Here's how the part is built. I have some questions about the finished solid (model axes, mm). Face numbers are marked on the shaded views. Round coordinates to 2 decimals unless told otherwise and drop trailing zeros. Write each loop counter-clockwise with the first axis right and the second up, starting at its lowest first coordinate (ties: lowest second). Pieces come first, ordered by that corner, then holes. Notation, with made-up numbers: (69.5, -15.5) -> (93.5, -15.5) arc R38 cw to (93.5, 22.5) -> close; hole circle Ø2 at (-26, -6). An arc over 180 degrees is marked (long way). Answer as CSV lines item,"result".
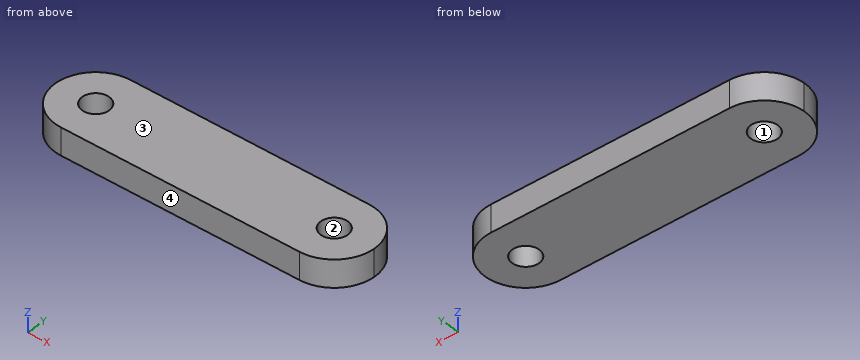
```python
from build123d import *

# Parameters (mm, degrees)
F1_DEPTH = 10
F2_R     = 5
F3_DEPTH = 25


with BuildPart() as f1:
    # F0 (on Top) → F1 (new body)
    with BuildSketch(Plane.XY):
        with BuildLine():
            ThreePointArc((60, 0), (55.606602, 10.606602), (45, 15))
            Line((45, 15), (-45, 15))
            ThreePointArc((-45, 15), (-55.606602, 10.606602), (-60, 0))
            ThreePointArc((-60, 0), (-55.606602, -10.606602), (-45, -15))
            Line((-45, -15), (45, -15))
            ThreePointArc((45, -15), (55.606602, -10.606602), (60, 0))
        make_face()
    extrude(amount=F1_DEPTH)

    # F2 (on face) → F3 (cut)
    with BuildSketch(Plane.XY.offset(10)):
        with Locations((-45, 0)):
            Circle(F2_R)
        with Locations((45, 0)):
            Circle(F2_R)
    extrude(amount=-F3_DEPTH, mode=Mode.SUBTRACT)


solid = f1.part
```
1. Suppose I cut it at A-A on z = 6.5. Please give me the cut outline in (x, y).
Numbers:
outline,"(-60, 0) arc R15 ccw to (-45, -15) -> (45, -15) arc R15 ccw to (60, 0) arc R15 ccw to (45, 15) -> (-45, 15) arc R15 ccw to start; hole circle Ø10 at (-45, 0); hole circle Ø10 at (45, 0)"
2. For pin 1 Ø3 at (y, z) = (-2.5, 6.5) entering from +X; pin 2 Ø8 at (x, y) = (-44, 1.5) entering from +Z; pin 3 Ø3 at (y, z) = (-4.5, 7) entering from -X, each with a flat end and sliding along its axis, tell me the tip position at first contact or that it passes through.
Numbers:
pin 1,"stops at x = 59.97"
pin 2,"stops at z = 10"
pin 3,"stops at x = -59.7"
3. Suppose I cut it at C-C on y = 9. Please give me the cut outline in (x, z).
Numbers:
outline,"(-57, 0) -> (57, 0) -> (57, 10) -> (-57, 10) -> close"
4. Suppose I cut it at B-B on y = -3.5. Please give me the cut outline in (x, z).
Numbers:
outline,"(-59.59, 0) -> (-48.57, 0) -> (-48.57, 10) -> (-59.59, 10) -> close; (-41.43, 0) -> (41.43, 0) -> (41.43, 10) -> (-41.43, 10) -> close; (48.57, 0) -> (59.59, 0) -> (59.59, 10) -> (48.57, 10) -> close"
5. If I drill on line 1 (Y direction, x = -45, z = 3.75); line 2 (X direction, y = -3.5, z = 8.75); line 3 (Y direction, x = 46.5, z = 4.25), over which ranges is the centre line in solid material (lowest first)?
Numbers:
line 1,"y = -15 to -5, 5 to 15"
line 2,"x = -59.59 to -48.57, -41.43 to 41.43, 48.57 to 59.59"
line 3,"y = -14.92 to -4.77, 4.77 to 14.92"
6. If we mould it in two halves opening along Y, with no side actions, what happens to the marked faces 1, 2, 3 and 4? For each: released by +Y, released by -Y, zero draft, split by the parting line, or undercut.
Numbers:
face 1,"undercut"
face 2,"undercut"
face 3,"zero draft"
face 4,"released by -Y"
